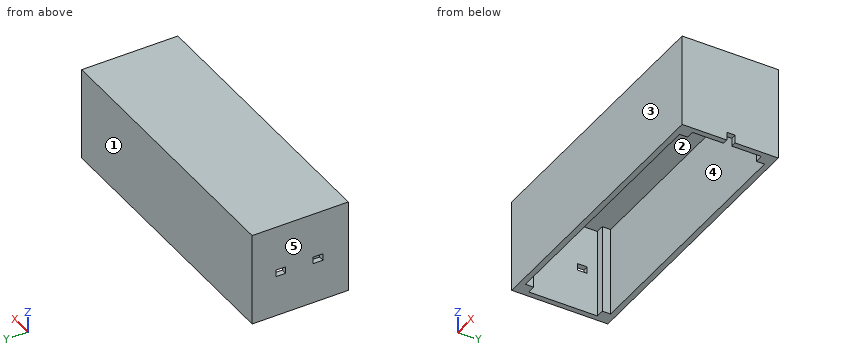
from build123d import *

# Parameters (mm, degrees)
SKETCH006_W     = 207
SKETCH006_H     = 70
PAD002_DEPTH    = 68
POCKET_DEPTH    = 65
SKETCH_W        = 7
SKETCH_H        = 5
POCKET001_DEPTH = 20
SKETCH008_W     = 6
SKETCH008_H     = 6
POCKET002_DEPTH = 10


with BuildPart() as part:
    # Sketch006 → Pad002 (new body)
    with BuildSketch(Plane.XY):
        with Locations((28.19796, -0.538714)):
            Rectangle(SKETCH006_W, SKETCH006_H)
    extrude(amount=PAD002_DEPTH)

    # Sketch007 (on Face5 of Pad002) → Pocket (cut)
    with BuildSketch(Plane(origin=(0, 0, 0), x_dir=(1, 0, 0), z_dir=(0, 0, -1))):
        Polygon((-65.30204, 31.538714), (-65.30204, 25.538714), (-71.30204, 25.538714), (-71.30204, -24.461286), (-65.30204, -24.461286), (-65.30204, -30.461286), (121.69796, -30.461286), (121.69796, -24.461286), (127.69796, -24.461286), (127.69796, 25.538714), (121.69796, 25.538714), (121.69796, 31.538714), align=None)
    extrude(amount=-POCKET_DEPTH, mode=Mode.SUBTRACT)

    # Sketch (on Face4 of Pad002) → Pocket001 (cut)
    with BuildSketch(Plane(origin=(-75.30204, 0, 0), x_dir=(0, -1, 0), z_dir=(-1, 0, 0))):
        with Locations((-13.5, 32.5)):
            Rectangle(SKETCH_W, SKETCH_H)
        with Locations((13.5, 32.5)):
            Rectangle(SKETCH_W, SKETCH_H)
    extrude(amount=-POCKET001_DEPTH, mode=Mode.SUBTRACT)

    # Sketch008 (on Face2 of Pad002) → Pocket002 (cut)
    with BuildSketch(Plane.YZ.offset(131.69796)):
        with Locations((0, 3)):
            Rectangle(SKETCH008_W, SKETCH008_H)
    extrude(amount=-POCKET002_DEPTH, mode=Mode.SUBTRACT)


solid = part.part
The listing builds one solid part. Answer for the finished solid, in the listing's coordinates (mm). Face numbers are marked on the shaded views. A direction names the side the tool comes from. Give positions to 0.01 mm unless a question says otherwise; leave off trailing zeros. Write each loop counter-clockwise with the first axis right and the second up, starting at its lowest first coordinate (ties: lowest second). Pieces come first, ordered by that corner, then holes.
Item 1: Flat-ended cylindrical pins translate along their axes: P1, Ø3, axis at x = 17.5, y = 17, coming from the -Z side; P2, Ø3, axis at x = -73.5, y = -13.5, coming from the -Z side. Find the tip coordinate at first contact, or state that the pin passes through.
Item 2: Find the intervals of material crossed by line 1 along Y through (x, z) = (9, 61); line 2 along X through (y, z) = (3, 43.5); line 3 along Y through (x, z) = (-66, 51.5), in increasing order.
Item 3: Section D-D, the plane y = 26.5 is taken. Write down the section's boundary in (x, z), plus the area to 3 significant figures.
Item 4: Which of the six approach directions +Z, -Z, +X, -X, +Y, -Y give full straight-line access (tool end or side, diameter ignored) to the marked faces 4 and 5?
Item 5: Determine the mould class of the marked faces 1, 2 and 3 for opening direction Y: released by +Y, released by -Y, zero draft, split by the parting line, or undercut.
Item 6: Section C-C, the plane x = 113 is taken. Write down the section's boundary in (y, z), plus the area to 3 significant figures.
Item 7: Section B-B, the plane y = 14 is taken. Write down the section's boundary in (x, z).
Item 8: Section A-A, the plane z = 41 is taken. Write down the section's boundary in (x, y), plus the area to 3 significant figures.
Completed:
1. P1: stops at z = 65
1. P2: stops at z = 0
2. line 1: y = -35.54 to -31.54, 30.46 to 34.46
2. line 2: x = -75.3 to -71.3, 127.7 to 131.7
2. line 3: y = -35.54 to -25.54, 24.46 to 34.46
3. outline: (-75.3, 0) - (-65.3, 0) - (-65.3, 65) - (121.7, 65) - (121.7, 0) - (131.7, 0) - (131.7, 68) - (-75.3, 68) - close
3. area: 1,920 mm2
4. face 4: -Z
4. face 5: +Z, -Z, -X, +Y, -Y
5. face 1: released by +Y
5. face 2: undercut
5. face 3: released by -Y
6. outline: (-35.54, 0) - (-31.54, 0) - (-31.54, 65) - (30.46, 65) - (30.46, 0) - (34.46, 0) - (34.46, 68) - (-35.54, 68) - close
6. area: 730 mm2
7. outline: (-75.3, 0) - (-71.3, 0) - (-71.3, 30) - (-75.3, 30) - close; (-75.3, 35) - (-71.3, 35) - (-71.3, 65) - (127.7, 65) - (127.7, 0) - (131.7, 0) - (131.7, 68) - (-75.3, 68) - close
8. outline: (-75.3, -35.54) - (131.7, -35.54) - (131.7, 34.46) - (-75.3, 34.46) - close; hole (-71.3, -25.54) - (-65.3, -25.54) - (-65.3, -31.54) - (121.7, -31.54) - (121.7, -25.54) - (127.7, -25.54) - (127.7, 24.46) - (121.7, 24.46) - (121.7, 30.46) - (-65.3, 30.46) - (-65.3, 24.46) - (-71.3, 24.46) - close
8. area: 2,300 mm2
